Geometry: final body of the model. Coordinates: model frame, mm. A direction names the side the tool comes from. Round coordinates to 2 decimals unless told otherwise and drop trailing zeros. Loops run counter-clockwise (first coordinate to the right, second up) from the corner with the lowest first, then second, coordinate; pieces in that order, holes last. Notation, with made-up numbers: M -16.75,86.5 L 6.25,86.5 A15 cw 6.25,104.5 Z; hole C 77,78.5 d2. An arc over 180 degrees is marked long. Answer as a JSON object with one key per item and string values.
from build123d import *

# Parameters (mm, degrees)
SKETCH1_W           = 42.5
SKETCH1_H           = 66
BOSS_EXTRUDE1_DEPTH = 5
SKETCH2_R           = 9
SKETCH2_R_2         = 1.5
CUT_EXTRUDE1_DEPTH  = 40.56718969
SKETCH3_W           = 28
SKETCH3_H           = 28
CUT_EXTRUDE2_DEPTH  = 40.56718969
SKETCH4_R           = 2
CUT_EXTRUDE3_DEPTH  = 40.56718969


with BuildPart() as part:
    # Sketch1 → Boss-Extrude1 (new body)
    with BuildSketch(Plane.XY):
        Rectangle(SKETCH1_W, SKETCH1_H)
    extrude(amount=BOSS_EXTRUDE1_DEPTH)

    # Sketch2 → Cut-Extrude1 (cut, through all)
    with BuildSketch(Plane.XY.offset(5)):
        with Locations((0, 16.5)):
            Circle(SKETCH2_R)
        with Locations((0, 27.5)):
            Circle(SKETCH2_R_2)
        with Locations((11, 16.5)):
            Circle(SKETCH2_R_2)
        with Locations((-11, 16.5)):
            Circle(SKETCH2_R_2)
        with Locations((0, 5.5)):
            Circle(SKETCH2_R_2)
    extrude(amount=-CUT_EXTRUDE1_DEPTH, mode=Mode.SUBTRACT)

    # Sketch3 → Cut-Extrude2 (cut, through all)
    with BuildSketch(Plane.XY.offset(5)):
        with Locations((0, -16.5)):
            Rectangle(SKETCH3_W, SKETCH3_H)
    extrude(amount=-CUT_EXTRUDE2_DEPTH, mode=Mode.SUBTRACT)

    # Sketch4 → Cut-Extrude3 (cut, through all)
    with BuildSketch(Plane.XY.offset(5)):
        with Locations((-17.75, 29.25)):
            Circle(SKETCH4_R)
        with Locations((17.75, 29.25)):
            Circle(SKETCH4_R)
        with Locations((-17.75, -29.25)):
            Circle(SKETCH4_R)
        with Locations((17.75, -29.25)):
            Circle(SKETCH4_R)
    extrude(amount=-CUT_EXTRUDE3_DEPTH, mode=Mode.SUBTRACT)


solid = part.part
1) Section query D-D (y = 16.5). Return the cut outline in (x, z), and give its area (3 significant figures).
Results:
{"outline": "M -21.25,0 L -12.5,0 L -12.5,5 L -21.25,5 Z; M -9.5,0 L -9,0 L -9,5 L -9.5,5 Z; M 9,0 L 9.5,0 L 9.5,5 L 9,5 Z; M 12.5,0 L 21.25,0 L 21.25,5 L 12.5,5 Z", "area": "92.5 mm2"}
2) Section query B-B (x = 0). Return the cut outline in (y, z), and give its area (3 significant figures).
Results:
{"outline": "M -33,0 L -30.5,0 L -30.5,5 L -33,5 Z; M -2.5,0 L 4,0 L 4,5 L -2.5,5 Z; M 7,0 L 7.5,0 L 7.5,5 L 7,5 Z; M 25.5,0 L 26,0 L 26,5 L 25.5,5 Z; M 29,0 L 33,0 L 33,5 L 29,5 Z", "area": "70.0 mm2"}
3) Section query C-C (x = 11). Return the cut outline in (y, z).
Results:
{"outline": "M -33,0 L -30.5,0 L -30.5,5 L -33,5 Z; M -2.5,0 L 15,0 L 15,5 L -2.5,5 Z; M 18,0 L 33,0 L 33,5 L 18,5 Z"}
4) Pull-direction query (X, two-part tool) for faces 3 (the cylindrical face through (0, 29, 3)), 4 (the flat face through (21.25, 0, 2)), 5 (the flat face through (0, -33, 2)); classes: +X half, -X half, draft (parallel to the pull), parting line (faces both ways), or undercut.
Results:
{"face 3": "undercut", "face 4": "+X half", "face 5": "draft"}
5) Section query A-A (y = -8). Return the cut outline in (x, z).
Results:
{"outline": "M -21.25,0 L -14,0 L -14,5 L -21.25,5 Z; M 14,0 L 21.25,0 L 21.25,5 L 14,5 Z"}
6) Pin query (flat end, axial travel): P1, Ø1.8, axis at x = 0, y = 27.5, coming from the +Z side; P2, Ø12, axis at x = 1, y = 21.5, coming from the +Z side. Return the tip coordinate at first contact, or that it passes through.
Results:
{"P1": "through", "P2": "z = 5"}
7) Ray query, line 1 (Y direction, x = 17.75, z = 1.45); line 2 (Y direction, x = 0, z = 1.1); line 3 (X direction, y = -29, z = 3.8). Return the intervals inside material, ascending.
Results:
{"line 1": "-33 to -31.25, -27.25 to 27.25, 31.25 to 33", "line 2": "-33 to -30.5, -2.5 to 4, 7 to 7.5, 25.5 to 26, 29 to 33", "line 3": "-21.25 to -19.73, -15.77 to -14, 14 to 15.77, 19.73 to 21.25"}
8) Reachability of faces 1 (the flat face through (0, -2.5, 3)), 2 (the flat face through (-5, 8, 5)) from +Z, -Z, +X, -X, +Y, -Y: full face, straight path, thin tool, end or side. Return the list, or none.
Results:
{"face 1": "+Z, -Z", "face 2": "+Z, +X, -X, +Y, -Y"}
